Geometry: final body of the model. Coordinates: model frame, mm. Round coordinates to 2 decimals unless told otherwise and drop trailing zeros. Loops run counter-clockwise (first coordinate to the right, second up) from the corner with the lowest first, then second, coordinate; pieces in that order, holes last. Notation, with made-up numbers: M -18,-32 L 31,-32 A23 ccw 31,-2 Z; hole C 8.5,44.5 d10. An arc over 180 degrees is marked long. Return JSON: item names as keys, results as strings.
from build123d import *

# Parameters (mm, degrees)
SALIENTE_EXTRUIR1_DEPTH = 12.7
CROQUIS2_R              = 6.35
CORTAR_EXTRUIR1_DEPTH   = 13.7


with BuildPart() as part:
    # Croquis1 → Saliente-Extruir1 (new body)
    with BuildSketch(Plane(origin=(0, 0, 0), x_dir=(1, 0, 0), z_dir=(0, 1, 0))):
        with BuildLine():
            Line((-109, -140), (109, -140))
            ThreePointArc((109, -140), (130.920310217, -130.920310217), (140, -109))
            Line((140, -109), (140, 109))
            ThreePointArc((140, 109), (130.920310217, 130.920310217), (109, 140))
            Line((109, 140), (-109, 140))
            ThreePointArc((-109, 140), (-130.920310217, 130.920310217), (-140, 109))
            Line((-140, 109), (-140, -109))
            ThreePointArc((-140, -109), (-130.920310217, -130.920310217), (-109, -140))
        make_face()
    extrude(amount=SALIENTE_EXTRUIR1_DEPTH)

    # Croquis2 → Cortar-Extruir1 (cut, through all)
    with BuildSketch(Plane(origin=(0, 12.7, 0), x_dir=(1, 0, 0), z_dir=(0, 1, 0))):
        with Locations((109, 109)):
            Circle(CROQUIS2_R)
        with Locations((109, -109)):
            Circle(CROQUIS2_R)
        with Locations((-109, -109)):
            Circle(CROQUIS2_R)
        with Locations((-109, 109)):
            Circle(CROQUIS2_R)
    extrude(amount=-CORTAR_EXTRUIR1_DEPTH, mode=Mode.SUBTRACT)


solid = part.part
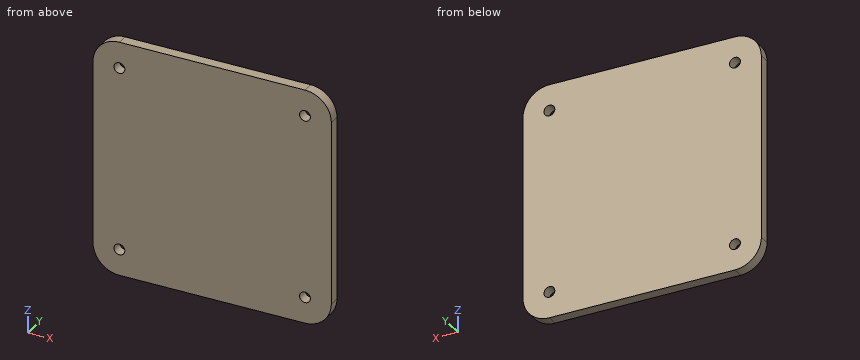
Q1. Section query B-B (z = -122). Output: boundary loops of the cut face in (x, y).
Determined:
{"outline": "M -137.14,0 L 137.14,0 L 137.14,12.7 L -137.14,12.7 Z"}
Q2. Material intervals for L1, parallel to Z at x = -109, y = 9.25; L2, parallel to Z at x = -120.5, y = 3.25, sorted ascending.
Determined:
{"L1": "z = -140 to -115.35, -102.65 to 102.65, 115.35 to 140", "L2": "z = -137.79 to 137.79"}
Q3. Pin query (flat end, axial travel): pin 1 (20.5 mm diameter, centred on x = 109, z = -109, fed in from -Y). Return the tip coordinate at first contact, or that it passes through.
Determined:
{"pin 1": "stops at y = 0"}
Q4. Section query A-A (y = 8.75). Output: boundary loops of the cut face in (x, z), plus the area to 3 significant figures.
Determined:
{"outline": "M -140,-109 A31 ccw -109,-140 L 109,-140 A31 ccw 140,-109 L 140,109 A31 ccw 109,140 L -109,140 A31 ccw -140,109 Z; hole C -109,-109 d12.7; hole C -109,109 d12.7; hole C 109,-109 d12.7; hole C 109,109 d12.7", "area": "77,100 mm^2"}
